```python
from build123d import *

# Parameters (mm, degrees)
CROQUIS1_W              = 40
CROQUIS1_H              = 45
SALIENTE_EXTRUIR1_DEPTH = 8
CROQUIS2_W              = 32.5
CROQUIS2_H              = 1.3
CORTAR_EXTRUIR1_DEPTH   = 6.6
CROQUIS3_R              = 15
CORTAR_EXTRUIR2_DEPTH   = 10
CHAFL_N1_SIZE           = 2
CROQUIS4_W              = 28.5
CROQUIS4_H              = 28
CORTAR_EXTRUIR3_DEPTH   = 6.6
CROQUIS6_R              = 2.75
CORTAR_EXTRUIR4_DEPTH   = 16.6
CROQUIS7_R              = 1.65
CORTAR_EXTRUIR5_DEPTH   = 16.6
CROQUIS8_R              = 4
CORTAR_EXTRUIR6_DEPTH   = 4
CROQUIS9_W              = 20
CROQUIS9_H              = 6.6
CORTAR_EXTRUIR7_DEPTH   = 4
REDONDEO1_R             = 1
REDONDEO2_R             = 2
REDONDEO3_R             = 1
REDONDEO4_R             = 3
REDONDEO5_R             = 0.5
REDONDEO6_R             = 0.5


with BuildPart() as part:
    # Croquis1 → Saliente-Extruir1 (new body)
    with BuildSketch(Plane.XY):
        Rectangle(CROQUIS1_W, CROQUIS1_H)
    extrude(amount=SALIENTE_EXTRUIR1_DEPTH)

    # Croquis2 → Cortar-Extruir1 (cut)
    with BuildSketch(Plane.XY.offset(8)):
        with Locations((0, -21.15)):
            Rectangle(CROQUIS2_W, CROQUIS2_H)
    extrude(amount=-CORTAR_EXTRUIR1_DEPTH, mode=Mode.SUBTRACT)

    # Croquis3 → Cortar-Extruir2 (cut)
    with BuildSketch(Plane.XY.offset(8)):
        with Locations((-30, -6.5)):
            Circle(CROQUIS3_R)
        with Locations((30, -6.5)):
            Circle(CROQUIS3_R)
    extrude(amount=-CORTAR_EXTRUIR2_DEPTH, mode=Mode.SUBTRACT)

    # Chaflán1
    chafl_n1_edges = [part.edges().sort_by_distance(p)[0] for p in [
        (-15, -6.5, 0),
        (15, -6.5, 0),
    ]]
    chamfer(chafl_n1_edges, length=CHAFL_N1_SIZE)

    # Croquis4 → Cortar-Extruir3 (cut)
    with BuildSketch(Plane.XY.offset(8)):
        with Locations((0, -6.5)):
            Rectangle(CROQUIS4_W, CROQUIS4_H)
    extrude(amount=-CORTAR_EXTRUIR3_DEPTH, mode=Mode.SUBTRACT)

    # Croquis6 → Cortar-Extruir4 (cut)
    with BuildSketch(Plane(origin=(0, 22.5, 0), x_dir=(1, 0, 0), z_dir=(0, 1, 0))):
        with Locations((0, -8)):
            Circle(CROQUIS6_R)
    extrude(amount=-CORTAR_EXTRUIR4_DEPTH, mode=Mode.SUBTRACT)

    # Croquis7 → Cortar-Extruir5 (cut)
    with BuildSketch(Plane.XY.offset(8)):
        with Locations((13, 15.5)):
            Circle(CROQUIS7_R)
        with Locations((-13, 15.5)):
            Circle(CROQUIS7_R)
    extrude(amount=-CORTAR_EXTRUIR5_DEPTH, mode=Mode.SUBTRACT)

    # Croquis8 → Cortar-Extruir6 (cut)
    with BuildSketch(Plane(origin=(0, 0, 0), x_dir=(-1, 0, 0), z_dir=(0, 0, -1))):
        with Locations((13, 15.5)):
            Circle(CROQUIS8_R)
        with Locations((-13, 15.5)):
            Circle(CROQUIS8_R)
    extrude(amount=-CORTAR_EXTRUIR6_DEPTH, mode=Mode.SUBTRACT)

    # Croquis9 → Cortar-Extruir7 (cut)
    with BuildSketch(Plane(origin=(0, -22.5, 0), x_dir=(-1, 0, 0), z_dir=(0, -1, 0))):
        with Locations((0, -4.7)):
            Rectangle(CROQUIS9_W, CROQUIS9_H)
    extrude(amount=-CORTAR_EXTRUIR7_DEPTH, mode=Mode.SUBTRACT)

    # Redondeo1
    redondeo1_edges = [part.edges().sort_by_distance(p)[0] for p in [
        (0, 22.5, 5.25),
    ]]
    fillet(redondeo1_edges, radius=REDONDEO1_R)

    # Redondeo2
    redondeo2_edges = [part.edges().sort_by_distance(p)[0] for p in [
        (-20, 22.5, 4),
        (20, 22.5, 4),
    ]]
    fillet(redondeo2_edges, radius=REDONDEO2_R)

    # Redondeo3
    redondeo3_edges = [part.edges().sort_by_distance(p)[0] for p in [
        (20, -22.5, 4),
        (-20, -22.5, 4),
    ]]
    fillet(redondeo3_edges, radius=REDONDEO3_R)

    # Redondeo4
    redondeo4_edges = [part.edges().sort_by_distance(p)[0] for p in [
        (0, 7.5, 5.25),
    ]]
    fillet(redondeo4_edges, radius=REDONDEO4_R)

    # Redondeo5
    redondeo5_edges = [part.edges().sort_by_distance(p)[0] for p in [
        (14.25, -20.5, 4.7),
        (-14.25, -20.5, 4.7),
    ]]
    fillet(redondeo5_edges, radius=REDONDEO5_R)

    # Redondeo6
    redondeo6_edges = [part.edges().sort_by_distance(p)[0] for p in [
        (-14.25, 7.5, 4.7),
        (14.25, 7.5, 4.7),
    ]]
    fillet(redondeo6_edges, radius=REDONDEO6_R)


solid = part.part
```
Here's how the part is built. I have some questions about the finished solid (model axes, mm). A direction names the side the tool comes from. Coordinates: 2 decimals unless noted, no trailing zeros. Loops run counter-clockwise (first coordinate to the right, second up) from the corner with the lowest first, then second, coordinate; pieces in that order, holes last. Notation, with made-up numbers: (76.5, -19.5) - (120.5, -19.5) arc R28 ccw to (120.5, 18.5) - close; hole circle Ø6 at (-22.5, 23). An arc over 180 degrees is marked (long way). Return JSON: item names as keys, results as strings. Group by question number.
Item 1: On a 3-axis mill with a long thin cutter (end or side, diameter ignored), from which of +Z, -Z, +X, -X, +Y, -Y can I reach the whole of each face in a straight line? I mean faces 4 (the face through (0, 7.5, 2)), 5 (the face through (-15, -6.7, 5)), 6 (the face through (-15, 16, 4)). Say none if no direction works.
Item 2: If we section it at B-B on x = 0: Write out the boundary of the cut face in (y, z).
Item 3: We'd pull the mould along Y, two halves only. Please class faces 1 (the face through (0, 0, 0)), 2 (the face through (-19.4, 21.93, 4.06)), 3 (the face through (-12.479, 19.466, 1.972)): +Y half, -Y half, draft (parallel to the pull), parting line (faces both ways), or undercut.
Item 4: Will these pins go through, and if not, where does the flat tip stop? P1, Ø3.5, axis at x = -3.5, z = 6, coming from the -Y side; P2, Ø3, axis at y = -1, z = 6.5, coming from the -X side; P3, Ø1.5, axis at y = -16.5, z = 4, coming from the +X side; P4, Ø2.5, axis at x = -13, y = 15.5, coming from the +Z side.
Item 5: If we section it at A-A on y = 15.5: Write out the boundary of the cut face in (x, z).
Item 6: I need wall thicknesses on line 1 (Y direction, x = 13, z = 1.45); line 2 (Y direction, x = -13, z = 5.45); line 3 (X direction, y = 7, z = 4.75). Which ranges of each line are inside material? Lowest first, please. Write a range as from..to.
Item 7: If we section it at C-C on x = -10.5: Write out the boundary of the cut face in (y, z).
Calculated:
{
 "1": {"face 4": "+Z", "face 5": "+Z, -Z, -X", "face 6": "-Z"},
 "2": {"outline": "(-22.5, 0) - (22.5, 0) - (22.5, 4.25) arc R1 ccw to (21.5, 5.25) - (10.5, 5.25) arc R3 ccw to (7.5, 2.25) - (7.5, 1.4) - (-22.5, 1.4) - close"},
 "3": {"face 1": "draft", "face 2": "+Y half", "face 3": "undercut"},
 "4": {"P1": "stops at y = 7.5", "P2": "stops at x = -16.73", "P3": "stops at x = 19.54", "P4": "passes through"},
 "5": {"outline": "(-20, 0) - (-17, 0) - (-17, 4) - (-14.65, 4) - (-14.65, 8) - (-20, 8) - close; (-11.35, 4) - (-9, 4) - (-9, 0) - (9, 0) - (9, 4) - (11.35, 4) - (11.35, 8) - (2.75, 8) arc R2.75 cw to (-2.75, 8) - (-11.35, 8) - close; (14.65, 4) - (17, 4) - (17, 0) - (20, 0) - (20, 8) - (14.65, 8) - close"},
 "6": {"line 1": "y = -22.5..-21.8, 7.5..11.5, 19.5..22.5", "line 2": "y = -22.5..-21.8, 7.5..13.85, 17.15..22.5", "line 3": "x = -20..-14.25, 14.25..20"},
 "7": {"outline": "(-22.5, 0) - (12.38, 0) - (12.38, 4) - (18.62, 4) - (18.62, 0) - (22.5, 0) - (22.5, 8) - (7.5, 8) - (7.5, 1.4) - (-21.8, 1.4) - (-21.8, 8) - (-22.5, 8) - close"}
}
